Verification items for the finished model (mm, model axes). Face numbers are marked on the shaded views. A direction names the side the tool comes from. Give positions to 0.01 mm unless a question says otherwise; leave off trailing zeros. Write each loop counter-clockwise with the first axis right and the second up, starting at its lowest first coordinate (ties: lowest second). Pieces come first, ordered by that corner, then holes. Notation, with made-up numbers: M 32.5,-5.75 L 66.5,-5.75 A27 cw 66.5,18.25 Z; hole C 67.5,-16 d3. An arc over 180 degrees is marked long. Answer as a JSON object with one key per item and string values.
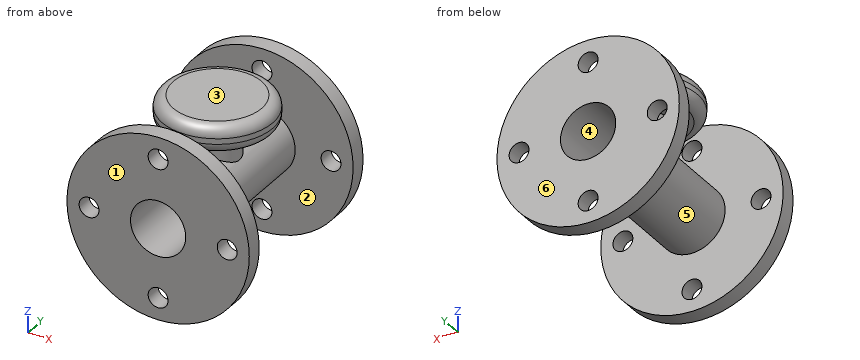
```python
from build123d import *

# Parameters (mm, degrees)
F0_R     = 30
F0_R_2   = 25
F1_DEPTH = 172
F2_R     = 82.5
F2_R_2   = 9
F2_R_3   = 30
F3_DEPTH = 15
F4_R     = 82.5
F4_R_2   = 9
F4_R_3   = 25
F5_DEPTH = 15
F6_R     = 20
F7_DEPTH = 50
F8_R     = 50
F8_R_2   = 20
F9_DEPTH = 25
F10_R    = 10


with BuildPart() as f1:
    # F0 (on Front) → F1 (new body)
    with BuildSketch(Plane.XZ):
        Circle(F0_R)
        Circle(F0_R_2, mode=Mode.SUBTRACT)
    extrude(amount=F1_DEPTH)

    # F2 (on face) → F3 (join)
    with BuildSketch(Plane(origin=(0, 0, 0), x_dir=(-1, 0, 0), z_dir=(0, 1, 0))):
        Circle(F2_R)
        with Locations((0, -62.5)):
            Circle(F2_R_2, mode=Mode.SUBTRACT)
        with Locations((-62.5, 0)):
            Circle(F2_R_2, mode=Mode.SUBTRACT)
        Circle(F2_R_3, mode=Mode.SUBTRACT)
        with Locations((62.5, 0)):
            Circle(F2_R_2, mode=Mode.SUBTRACT)
        with Locations((0, 62.5)):
            Circle(F2_R_2, mode=Mode.SUBTRACT)
    extrude(amount=-F3_DEPTH)

    # F4 (on face) → F5 (join)
    with BuildSketch(Plane.XZ.offset(172)):
        Circle(F4_R)
        with Locations((0, -62.5)):
            Circle(F4_R_2, mode=Mode.SUBTRACT)
        with Locations((-62.5, 0)):
            Circle(F4_R_2, mode=Mode.SUBTRACT)
        Circle(F4_R_3, mode=Mode.SUBTRACT)
        with Locations((62.5, 0)):
            Circle(F4_R_2, mode=Mode.SUBTRACT)
        with Locations((0, 62.5)):
            Circle(F4_R_2, mode=Mode.SUBTRACT)
    extrude(amount=-F5_DEPTH)

    # F6 (on Top) → F7 (join)
    with BuildSketch(Plane.XY):
        with Locations((0, -82.25701)):
            Circle(F6_R)
    extrude(amount=F7_DEPTH)

    # F8 (on face) → F9 (join)
    with BuildSketch(Plane.XY.offset(50)):
        with Locations((0, -82.25701)):
            Circle(F8_R)
        with Locations((0, -82.25701)):
            Circle(F8_R_2, mode=Mode.SUBTRACT)
        with Locations((0, -82.25701)):
            Circle(F8_R_2)
    extrude(amount=F9_DEPTH)

    # F10
    f10_edges = [f1.edges().sort_by_distance(p)[0] for p in [
        (-50, -82.25701, 75),
        (-50, -82.25701, 50),
    ]]
    fillet(f10_edges, radius=F10_R)


solid = f1.part
```
1) Release check for a two-part mould opening along Z. For the marked faces 3, 4, 5 and 6 record: pulls with the +Z half, pulls with the -Z half, needs draft (parallel to the pull), parting line crosses it, or undercut.
Completed:
{"face 3": "pulls with the +Z half", "face 4": "undercut", "face 5": "undercut", "face 6": "needs draft"}
2) Section check B-B on x = 61. Record the boundary of the cut face in (y, z), and give its area (3 significant figures).
Completed:
{"outline": "M -172,-55.55 L -157,-55.55 L -157,-8.87 L -172,-8.87 Z; M -172,8.87 L -157,8.87 L -157,55.55 L -172,55.55 Z; M -15,-55.55 L 0,-55.55 L 0,-8.87 L -15,-8.87 Z; M -15,8.87 L 0,8.87 L 0,55.55 L -15,55.55 Z", "area": "2,800 mm2"}
3) Section check C-C on z = -62.5. Record the boundary of the cut face in (x, y), and give its area (3 significant figures).
Completed:
{"outline": "M -53.85,-172 L -9,-172 L -9,-157 L -53.85,-157 Z; M -53.85,-15 L -9,-15 L -9,0 L -53.85,0 Z; M 9,-172 L 53.85,-172 L 53.85,-157 L 9,-157 Z; M 9,-15 L 53.85,-15 L 53.85,0 L 9,0 Z", "area": "2,690 mm2"}
4) Access from +Z, -Z, +X, -X, +Y, -Y to the whole of each face (thin tool, end or side, straight path). Record for the marked faces 1 and 2.
Completed:
{"face 1": "+Z, -Z, +X, -X, -Y", "face 2": "none"}
5) Go/stop test with flat-tipped pins: pin 1 (3 mm diameter, centred on x = 20.5, y = -114, fed in from -Z); pin 2 (6 mm diameter, centred on y = -31.5, z = -1.5, fed in from +X); pin 3 (14.5 mm diameter, centred on x = 0, z = 62.5, fed in from +Y); pin 4 (20.5 mm diameter, centred on x = 0, z = -62.5, fed in from -Y). Record where each tip stops, or that it passes through.
Completed:
{"pin 1": "stops at z = -23.22", "pin 2": "stops at x = 30", "pin 3": "stops at y = -32.26", "pin 4": "stops at y = -172"}
6) Section check D-D on z = 62.5. Record the boundary of the cut face in (x, y).
Completed:
{"outline": "M -53.85,-172 L -9,-172 L -9,-157 L -53.85,-157 Z; M -53.85,-15 L -9,-15 L -9,0 L -53.85,0 Z; C 0,-82.26 d100; M 9,-172 L 53.85,-172 L 53.85,-157 L 9,-157 Z; M 9,-15 L 53.85,-15 L 53.85,0 L 9,0 Z"}
7) Section check A-A on z = -19. Record the boundary of the cut face in (x, y).
Completed:
{"outline": "M -80.28,-172 L -16.25,-172 L -16.25,0 L -80.28,0 L -80.28,-15 L -23.22,-15 L -23.22,-157 L -80.28,-157 Z; M 16.25,-172 L 80.28,-172 L 80.28,-157 L 23.22,-157 L 23.22,-15 L 80.28,-15 L 80.28,0 L 16.25,0 Z"}
8) Thickness scan on L1, parallel to Z at x = 0, y = -6; L2, parallel to Z at x = 0, y = -43; L3, parallel to Y at x = -28.5, z = -36. Record the ranges inside material, lowest first.
Completed:
{"L1": "z = -82.5 to -71.5, -53.5 to -25, 25 to 53.5, 71.5 to 82.5", "L2": "z = -30 to -25, 25 to 30, 50 to 75", "L3": "y = -172 to -157, -15 to 0"}
